Verification items for this drawing (mm, ordinates from the low corner). Round coordinates to 2 decimals unless told otherwise and drop trailing zeros. Loops run counter-clockwise (first coordinate to the right, second up) from the corner with the lowest first, then second, coordinate; pieces in that order, holes last. Notation, with made-up numbers: (6, 76) - (30, 76) arc R17 ccw to (30, 90) - close; hole circle Ø6 at (80, 15). An arc over 180 degrees is marked (long way). Write item = value, one per line.
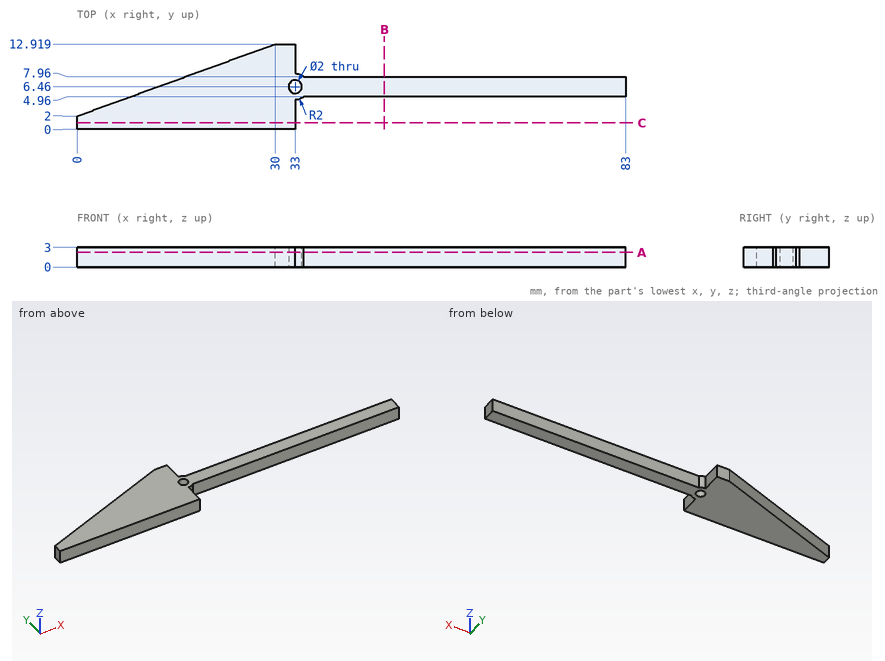
(1) Section check C-C (y = 1). Enter the section's corners in (x, z).
Answers follow:
outline = (0, 0) - (33, 0) - (33, 3) - (0, 3) - close
(2) Gauge pin test, flat ends, axial feed: pin 1 (0.9 mm diameter, centred on x = 54.5, z = 1.5, fed in from -Y); pin 2 (1 mm diameter, centred on x = 63.5, y = 3.5, fed in from -Z). Record the tip position at first contact, or that the pin passes through.
Answers follow:
pin_1 = 4.96
pin_2 = through
(3) Section check A-A (z = 2.25). Enter the section's corners in (x, y), then the cut area to 3 significant figures.
Answers follow:
outline = (0, 0) - (33, 0) - (33, 4.46) arc R2 ccw to (34.32, 4.96) - (83, 4.96) - (83, 7.96) - (34.32, 7.96) arc R2 ccw to (33, 8.46) - (33, 12.92) - (30, 12.92) - (0, 2) - close; hole circle Ø2 at (33, 6.46)
area = 410 mm²
(4) Scan lines: L1, parallel to X at y = 1.5, z = 1.85; L2, parallel to Y at x = 49.5, z = 1.8; L3, parallel to Y at x = 17, z = 1.7. Record each from-to range of solid material in increasing order. Write a range as [from, to].
Answers follow:
L1 = [0, 33]
L2 = [4.96, 7.96]
L3 = [0, 8.19]
(5) Section check B-B (x = 46.5). Enter the section's corners in (y, z).
Answers follow:
outline = (4.96, 0) - (7.96, 0) - (7.96, 3) - (4.96, 3) - close
